from build123d import *

# Parameters (mm, degrees)
SKETCH_1_R      = 2.1
EXTRUDE_1_DEPTH = 600


with BuildPart() as part:
    # 草图1 → 凸台-拉伸1 (new body)
    with BuildSketch(Plane.XY):
        with BuildLine():
            Line((-10, 19), (-10, 13.3))
            ThreePointArc((-10, 13.3), (-9.912132034, 13.087867966), (-9.7, 13))
            Line((-9.7, 13), (-8, 13))
            Line((-8, 13), (-8, 16))
            Line((-8, 16), (-7.060660172, 16))
            Line((-7.060660172, 16), (-4, 12.939339828))
            Line((-4, 12.939339828), (-4, 7.060660172))
            Line((-4, 7.060660172), (-7.060660172, 4))
            Line((-7.060660172, 4), (-8, 4))
            Line((-8, 4), (-8, 7))
            Line((-8, 7), (-9.7, 7))
            ThreePointArc((-9.7, 7), (-9.912132034, 6.912132034), (-10, 6.7))
            Line((-10, 6.7), (-10, -6.7))
            ThreePointArc((-10, -6.7), (-9.912132034, -6.912132034), (-9.7, -7))
            Line((-9.7, -7), (-8, -7))
            Line((-8, -7), (-8, -4))
            Line((-8, -4), (-7.060660172, -4))
            Line((-7.060660172, -4), (-4, -7.060660172))
            Line((-4, -7.060660172), (-4, -12.939339828))
            Line((-4, -12.939339828), (-7.060660172, -16))
            Line((-7.060660172, -16), (-8, -16))
            Line((-8, -16), (-8, -13))
            Line((-8, -13), (-9.7, -13))
            ThreePointArc((-9.7, -13), (-9.912132034, -13.087867966), (-10, -13.3))
            Line((-10, -13.3), (-10, -19))
            ThreePointArc((-10, -19), (-9.948683298, -19.316227766), (-9.8, -19.6))
            Line((-9.8, -19.6), (-3, -19.6))
            Line((-3, -19.6), (-3, -18))
            Line((-3, -18), (-6, -18))
            Line((-6, -18), (-6, -17.060660172))
            Line((-6, -17.060660172), (-2.939339828, -14))
            Line((-2.939339828, -14), (2.939339828, -14))
            Line((2.939339828, -14), (6, -17.060660172))
            Line((6, -17.060660172), (6, -18))
            Line((6, -18), (3, -18))
            Line((3, -18), (3, -19.6))
            Line((3, -19.6), (9.8, -19.6))
            ThreePointArc((9.8, -19.6), (9.948683298, -19.316227766), (10, -19))
            Line((10, -19), (10, -13.3))
            ThreePointArc((10, -13.3), (9.912132034, -13.087867966), (9.7, -13))
            Line((9.7, -13), (8, -13))
            Line((8, -13), (8, -16))
            Line((8, -16), (7.060660172, -16))
            Line((7.060660172, -16), (4, -12.939339828))
            Line((4, -12.939339828), (4, -7.060660172))
            Line((4, -7.060660172), (7.060660172, -4))
            Line((7.060660172, -4), (8, -4))
            Line((8, -4), (8, -7))
            Line((8, -7), (9.7, -7))
            ThreePointArc((9.7, -7), (9.912132034, -6.912132034), (10, -6.7))
            Line((10, -6.7), (10, 6.7))
            ThreePointArc((10, 6.7), (9.912132034, 6.912132034), (9.7, 7))
            Line((9.7, 7), (8, 7))
            Line((8, 7), (8, 4))
            Line((8, 4), (7.060660172, 4))
            Line((7.060660172, 4), (4, 7.060660172))
            Line((4, 7.060660172), (4, 12.939339828))
            Line((4, 12.939339828), (7.060660172, 16))
            Line((7.060660172, 16), (8, 16))
            Line((8, 16), (8, 13))
            Line((8, 13), (9.7, 13))
            ThreePointArc((9.7, 13), (9.912132034, 13.087867966), (10, 13.3))
            Line((10, 13.3), (10, 19))
            ThreePointArc((10, 19), (9.948683298, 19.316227766), (9.8, 19.6))
            Line((9.8, 19.6), (3, 19.6))
            Line((3, 19.6), (3, 18))
            Line((3, 18), (6, 18))
            Line((6, 18), (6, 17.060660172))
            Line((6, 17.060660172), (2.939339828, 14))
            Line((2.939339828, 14), (-2.939339828, 14))
            Line((-2.939339828, 14), (-6, 17.060660172))
            Line((-6, 17.060660172), (-6, 18))
            Line((-6, 18), (-3, 18))
            Line((-3, 18), (-3, 19.6))
            Line((-3, 19.6), (-9.8, 19.6))
            ThreePointArc((-9.8, 19.6), (-9.948683298, 19.316227766), (-10, 19))
        make_face()
        with Locations((0, -10)):
            Circle(SKETCH_1_R, mode=Mode.SUBTRACT)
        with Locations((0, 10)):
            Circle(SKETCH_1_R, mode=Mode.SUBTRACT)
        Polygon((-8, -2.5), (-6.439339828, -2.5), (-2.939339828, -6), (2.939339828, -6), (6.439339828, -2.5), (8, -2.5), (8, 2.5), (6.439339828, 2.5), (2.939339828, 6), (-2.939339828, 6), (-6.439339828, 2.5), (-8, 2.5), align=None, mode=Mode.SUBTRACT)
    extrude(amount=-EXTRUDE_1_DEPTH)


solid = part.part
Work out the finished part from the listing and answer in its coordinate system (mm). Round coordinates to 2 decimals unless told otherwise and drop trailing zeros. Use one line per item in the form item = value. Start each with the question number.
(1) Find section A-A on z = -177. Give the number of separate pieces and of enclosed holes in the cut face, and give its area (3 significant figures).
(2) Consider line 1 (Y direction, x = 0, z = -368); line 2 (X direction, y = 3, z = -69); line 3 (Y direction, x = -7.25, z = -209.5). Determine where each line is inside the solid, lowest interval first.
(3) Flat-ended cylindrical pins translate along their axes: P1, Ø4, axis at x = 0, y = 10, coming from the +Z side; P2, Ø12, axis at x = 1.5, y = -15.5, coming from the +Z side; P3, Ø1.5, axis at x = -2, z = -517, coming from the +Y side; P4, Ø1.5, axis at y = 9.5, z = -437.5, coming from the +X side. Find the tip coordinate at first contact, or state that the pin passes through.
Answer list:
q1.separate_pieces = 1
q1.enclosed_holes = 3
q1.area = 311 mm^2
q2.line_1 = -14 to -12.1, -7.9 to -6, 6 to 7.9, 12.1 to 14
q2.line_2 = -10 to -5.94, 5.94 to 10
q2.line_3 = -19.6 to -16, -4 to -2.5, 2.5 to 4, 16 to 19.6
q3.P1 = through
q3.P2 = 0
q3.P3 = 14
q3.P4 = 4
